Input: part model. Units: mm. Frame: model coordinates. Round coordinates to 2 decimals unless told otherwise and drop trailing zeros. Write each loop counter-clockwise with the first axis right and the second up, starting at its lowest first coordinate (ties: lowest second). Pieces come first, ordered by that corner, then holes. Notation, with made-up numbers: M 10.5,17.5 L 44.5,17.5 A28 ccw 44.5,47.5 Z; hole C 3,13 d5. An arc over 180 degrees is marked long. Answer as CSV lines item,"result". Start each with the question number.
```python
from build123d import *

# Parameters (mm, degrees)
SKETCH1_R           = 2.4765
BOSS_EXTRUDE1_DEPTH = 3.175


with BuildPart() as part:
    # Sketch1 → Boss-Extrude1 (new body)
    with BuildSketch(Plane.XY):
        Polygon((0, 0), (25.4, 0), (25.4, 50.8), (25.4, 101.6), (-25.4, 101.6), (-25.4, 50.8), (-25.4, 0), align=None)
        with Locations((12.7, 88.9)):
            Circle(SKETCH1_R, mode=Mode.SUBTRACT)
        with Locations((-12.7, 88.9)):
            Circle(SKETCH1_R, mode=Mode.SUBTRACT)
        with Locations((-12.7, 63.5)):
            Circle(SKETCH1_R, mode=Mode.SUBTRACT)
        with Locations((12.7, 63.5)):
            Circle(SKETCH1_R, mode=Mode.SUBTRACT)
        with Locations((12.7, 12.7)):
            Circle(SKETCH1_R, mode=Mode.SUBTRACT)
        with Locations((-12.7, 12.7)):
            Circle(SKETCH1_R, mode=Mode.SUBTRACT)
        with Locations((-12.7, 38.1)):
            Circle(SKETCH1_R, mode=Mode.SUBTRACT)
        with Locations((12.7, 38.1)):
            Circle(SKETCH1_R, mode=Mode.SUBTRACT)
    extrude(amount=BOSS_EXTRUDE1_DEPTH)


solid = part.part
```
Item 1: Cut plane D-D, the plane y = 62.5. Return loops of the section in (x, z) (3 decimals).
Item 2: Cut plane B-B, the plane x = 12.7. Return loops of the section in (y, z) (1 decimal).
Item 3: Pin query (flat end, axial travel): pin 1 Ø3 at (x, y) = (-4, 77.5) entering from -Z. Return the tip coordinate at first contact, or that it passes through.
Item 4: Cut plane C-C, the plane y = 12.7. Return loops of the section in (x, z) (1 decimal), plus the area to 3 significant figures.
Item 5: Line query: line 1 (Y direction, x = -12.7, z = 1.35); line 2 (Y direction, x = 10.5, z = 0.5). Output: solid intervals per line, ascending. Write a range as [from, to].
Item 6: Cut plane A-A, the plane z = 1.6. Give the number of separate pieces and of enclosed holes in the cut face, plus the area to 3 significant figures.
Item 7: Draft query along Y for faces 1 (the face through (12.378, 65.955, 1.565)), 2 (the face through (0, 0, 2)), 3 (the face through (0, 52, 0)), 4 (the face through (0, 101.6, 2)). Return one class per face: +Y half, -Y half, draft (parallel to the pull), parting line (faces both ways), or undercut.
Results list:
1,outline,"M -25.4,0 L -14.966,0 L -14.966,3.175 L -25.4,3.175 Z; M -10.434,0 L 10.434,0 L 10.434,3.175 L -10.434,3.175 Z; M 14.966,0 L 25.4,0 L 25.4,3.175 L 14.966,3.175 Z"
2,outline,"M 0,0 L 10.2,0 L 10.2,3.2 L 0,3.2 Z; M 15.2,0 L 35.6,0 L 35.6,3.2 L 15.2,3.2 Z; M 40.6,0 L 61,0 L 61,3.2 L 40.6,3.2 Z; M 66,0 L 86.4,0 L 86.4,3.2 L 66,3.2 Z; M 91.4,0 L 101.6,0 L 101.6,3.2 L 91.4,3.2 Z"
3,pin 1,"z = 0"
4,outline,"M -25.4,0 L -15.2,0 L -15.2,3.2 L -25.4,3.2 Z; M -10.2,0 L 10.2,0 L 10.2,3.2 L -10.2,3.2 Z; M 15.2,0 L 25.4,0 L 25.4,3.2 L 15.2,3.2 Z"
4,area,"130 mm²"
5,line 1,"[0, 10.22], [15.18, 35.62], [40.58, 61.02], [65.98, 86.42], [91.38, 101.6]"
5,line 2,"[0, 11.56], [13.84, 36.96], [39.24, 62.36], [64.64, 87.76], [90.04, 101.6]"
6,separate pieces,"1"
6,enclosed holes,"8"
6,area,"5,010 mm²"
7,face 1,"undercut"
7,face 2,"-Y half"
7,face 3,"draft"
7,face 4,"+Y half"
